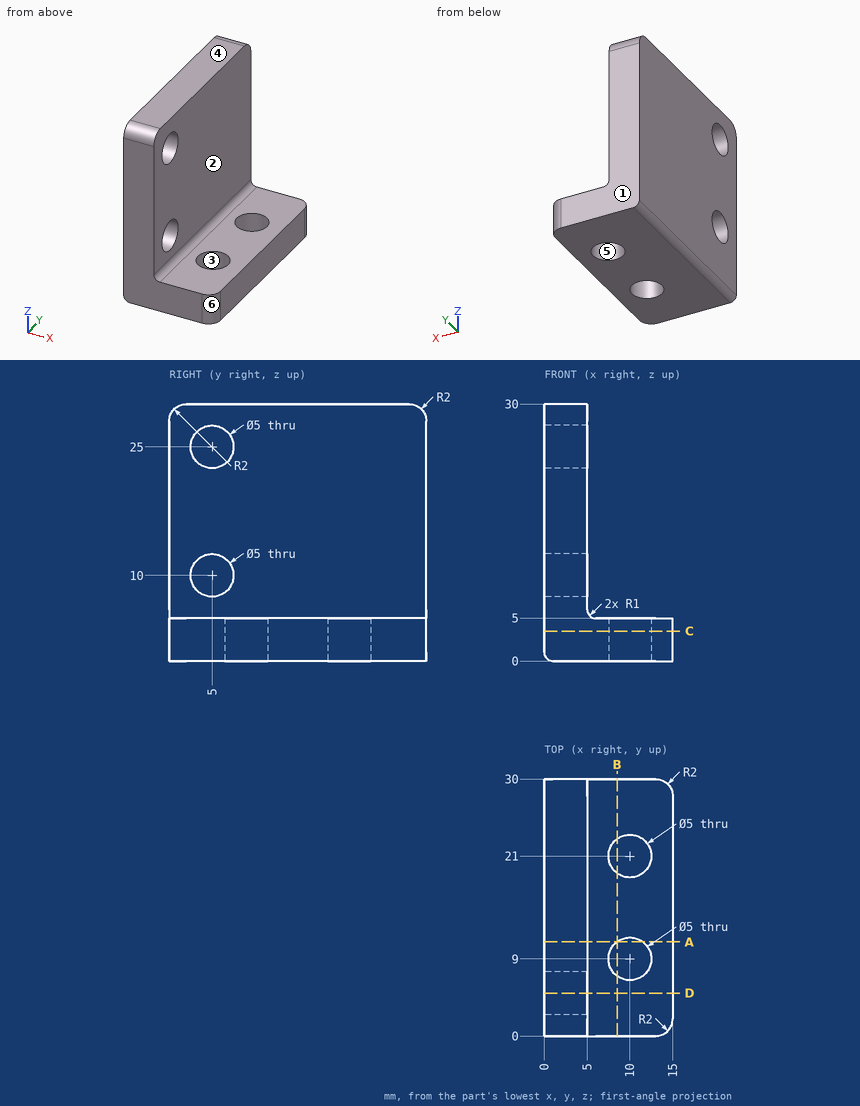
The drawing under review shows one solid part. Ordinate dimensions are in mm from its lowest x, y, z. A direction names the side the tool comes from. Coordinates: 2 decimals unless noted, no trailing zeros. Loops run counter-clockwise (first coordinate to the right, second up) from the corner with the lowest first, then second, coordinate; pieces in that order, holes last.
Item 1: Clearance check with flat-ended pins moving along their axes: pin 1 (6 mm diameter, centred on y = 4.5, z = 18, fed in from +X); pin 2 (4.5 mm diameter, centred on x = 10, y = 9, fed in from +Z); pin 3 (2.5 mm diameter, centred on x = 11, y = 18.5, fed in from +Z). State where each tip first meets the part, or that it passes through.
Completed:
pin 1: stops at x = 5
pin 2: passes through
pin 3: stops at z = 5
Item 2: Add section B-B (x = 8.5). Write out the cut boundary in (y, z).
Completed:
outline: (0, 0) - (7, 0) - (7, 5) - (0, 5) - close; (11, 0) - (19, 0) - (19, 5) - (11, 5) - close; (23, 0) - (30, 0) - (30, 5) - (23, 5) - close
Item 3: Add section A-A (y = 11). Write out the cut boundary in (x, z), and give its area (3 significant figures).
Completed:
outline: (0, 1) arc R1 ccw to (1, 0) - (8.5, 0) - (8.5, 5) - (6, 5) arc R1 cw to (5, 6) - (5, 30) - (0, 30) - close; (11.5, 0) - (15, 0) - (15, 5) - (11.5, 5) - close
area: 185 mm2
Item 4: For the marked faces 1 and 2, list the 3-axis set-ups (+Z, -Z, +X, -X, +Y, -Y) from which the entire face can be reached by the end or side of a thin tool; tool diameter is ignored.
Completed:
face 1: +Z, -Z, +X, -X, +Y
face 2: +Z, +X, +Y, -Y
Item 5: Add section D-D (y = 5). Write out the cut boundary in (x, z).
Completed:
outline: (0, 1) arc R1 ccw to (1, 0) - (15, 0) - (15, 5) - (6, 5) arc R1 cw to (5, 6) - (5, 7.5) - (0, 7.5) - close; (0, 12.5) - (5, 12.5) - (5, 22.5) - (0, 22.5) - close; (0, 27.5) - (5, 27.5) - (5, 30) - (0, 30) - close
Item 6: Wall thickness on L1, parallel to Y at x = 10, z = 2.2; L2, parallel to Z at x = 2.95, y = 5; L3, parallel to Y at x = 2.2, z = 25: over which ranges is each line inside the solid? List them lowest first.
Completed:
L1: y = 0 to 6.5, 11.5 to 18.5, 23.5 to 30
L2: z = 0 to 7.5, 12.5 to 22.5, 27.5 to 30
L3: y = 0 to 2.5, 7.5 to 30
Item 7: Draft analysis for pull direction Y (two halves, no side actions). For the marked faces 3, 4, 5 and 6, state which applies: pulls with the +Y half, pulls with the -Y half, needs draft (parallel to the pull), parting line crosses it, or undercut.
Completed:
face 3: undercut
face 4: needs draft
face 5: undercut
face 6: pulls with the -Y half
Item 8: Add section C-C (z = 3.5). Write out the cut boundary in (x, y).
Completed:
outline: (0, 0) - (13, 0) arc R2 ccw to (15, 2) - (15, 28) arc R2 ccw to (13, 30) - (0, 30) - close; hole circle Ø5 at (10, 9); hole circle Ø5 at (10, 21)
